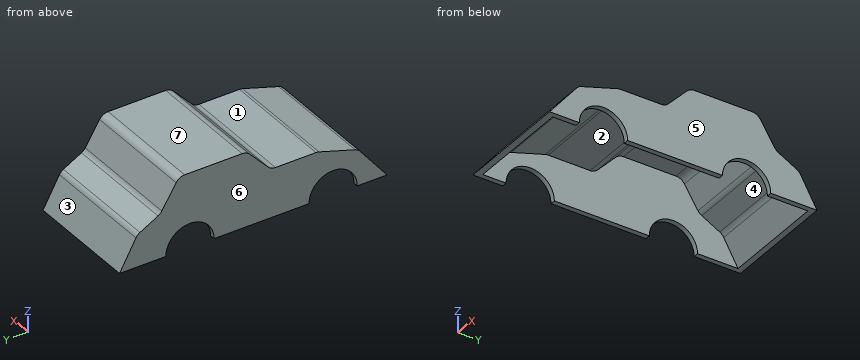
```python
from build123d import *

# Parameters (mm, degrees)
F1_DEPTH = 57
F2_T     = -2.5
F3_R     = 5
F4_R     = 5


with BuildPart() as f1:
    # F0 (on Right) → F1 (new body)
    with BuildSketch(Plane.YZ):
        with BuildLine():
            ThreePointArc((23.7267759775, 0), (35.7267759775, 12), (47.7267759775, 0))
            Line((47.7267759775, 0), (70.7267759775, 0))
            Line((70.7267759775, 0), (61.8750043213, 15.9051734954))
            Line((61.8750043213, 15.9051734954), (50.431035459, 22.1120696515))
            Line((50.431035459, 22.1120696515), (41.1206930876, 37))
            Line((41.1206930876, 37), (7.5646545738, 37))
            Line((7.5646545738, 37), (-4.6551725827, 24.0517258644))
            Line((-4.6551725827, 24.0517258644), (-27.737069875, 24.0517258644))
            Line((-27.737069875, 24.0517258644), (-47.9094833136, 17.8448278457))
            Line((-47.9094833136, 17.8448278457), (-62.2732240225, 0))
            Line((-62.2732240225, 0), (-47.4932240225, 0))
            ThreePointArc((-47.4932240225, 0), (-35.4932240225, 12), (-23.4932240225, 0))
            Line((-23.4932240225, 0), (23.7267759775, 0))
        make_face()
    extrude(amount=F1_DEPTH)

    # F2
    f2_openings = [f1.faces().sort_by_distance(p)[0] for p in [
        (28.5, 0.116776, 0),
        (28.5, -35.493224, 12),
        (28.5, 35.726776, 12),
        (28.5, 59.226776, 0),
        (28.5, -54.883224, 0),
    ]]
    offset(amount=F2_T, openings=f2_openings, kind=Kind.INTERSECTION)

    # F3
    f3_edges = [f1.edges().sort_by_distance(p)[0] for p in [
        (28.5, -47.909483, 17.844828),
        (28.5, -27.73707, 24.051726),
        (28.5, -4.655173, 24.051726),
        (28.5, 7.564655, 37),
        (28.5, 41.120693, 37),
        (28.5, 50.431035, 22.11207),
        (28.5, 61.875004, 15.905173),
    ]]
    fillet(f3_edges, radius=F3_R)

    # F4
    f4_edges = [f1.edges().sort_by_distance(p)[0] for p in [
        (28.5, -46.44224, 15.68062),
        (28.5, -27.361151, 21.551726),
        (28.5, -3.577006, 21.551726),
        (28.5, 8.642822, 34.5),
        (28.5, 39.735499, 34.5),
        (28.5, 48.660441, 20.228354),
        (28.5, 60.044051, 14.054195),
    ]]
    fillet(f4_edges, radius=F4_R)


solid = f1.part
```
Input: part model. Units: mm. Frame: model coordinates. Face numbers are marked on the shaded views. A direction names the side the tool comes from. Coordinates: 2 decimals unless noted, no trailing zeros. Write each loop counter-clockwise with the first axis right and the second up, starting at its lowest first coordinate (ties: lowest second). Pieces come first, ordered by that corner, then holes.
1) Section C-C on y = 55. Output: boundary loops of the cut face in (x, z), and give its area (3 significant figures).
2) Mould query, pull axis X, two halves, no side actions, for the marked faces 4, 5, 6 and 7. Classes: pulls with the +X half, pulls with the -X half, needs draft (parallel to the pull), parting line crosses it, or undercut.
3) Section B-B on z = 9. Output: boundary loops of the cut face in (x, y), and give its area (3 significant figures).
4) Pin query (flat end, axial travel): pin 1 Ø3 at (x, z) = (24.5, 11) entering from +Y; pin 2 Ø1 at (x, z) = (39.5, 16.5) entering from -Y; pin 3 Ø10 at (x, y) = (27, -41) entering from +Z. Return the tip coordinate at first contact, or that it passes through.
5) Material intervals for line 1 along X through (y, z) = (-22.5, 16); line 2 along Y through (x, z) = (55, 3.5); line 3 along Y through (x, z) = (15, 10.5), sorted ascending.
6) Set-up query: the marked faces 1, 2 and 3. Return all of +Z, -Z, +X, -X, +Y, -Y with unobstructed straight access to the full face (end or side cutting, diameter ignored); none if empty.
Check result:
1. outline: (0, 0) - (2.5, 0) - (2.5, 16.79) - (54.5, 16.79) - (54.5, 0) - (57, 0) - (57, 19.63) - (0, 19.63) - close
1. area: 246 mm2
2. face 4: undercut
2. face 5: pulls with the +X half
2. face 6: pulls with the -X half
2. face 7: needs draft
3. outline: (0, -55.03) - (57, -55.03) - (57, -43.43) - (54.5, -43.43) - (54.5, -51.82) - (2.5, -51.82) - (2.5, -43.43) - (0, -43.43) - close; (0, -27.56) - (2.5, -27.56) - (2.5, 27.79) - (0, 27.79) - close; (0, 43.66) - (2.5, 43.66) - (2.5, 62.86) - (54.5, 62.86) - (54.5, 43.66) - (57, 43.66) - (57, 65.72) - (0, 65.72) - close; (54.5, -27.56) - (57, -27.56) - (57, 27.79) - (54.5, 27.79) - close
3. area: 761 mm2
4. pin 1: stops at y = 65.44
4. pin 2: stops at y = -49.39
4. pin 3: stops at z = 21.51
5. line 1: x = 0 to 2.5, 54.5 to 57
5. line 2: y = -59.46 to -46.97, -24.01 to 24.25, 47.21 to 68.78
5. line 3: y = -53.82 to -50.61, 62.02 to 64.88
6. face 1: +Z, +X, -X, -Y
6. face 2: -Z
6. face 3: +Z, +X, -X, +Y
